```python
from build123d import *

# Parameters (mm, degrees)
SKETCH_1_R                   = 14
SKETCH_1_R_2                 = 2.75
EXTRUDE_1_DEPTH              = 27
CHAMFER_2_SIZE               = 1
HOLE_WIZARD_M5_4_D           = 5.5
HOLE_WIZARD_M5_4_CBORE_D     = 10
HOLE_WIZARD_M5_4_CBORE_DEPTH = 5.4
PATTERN_CIRCULAR_1_COUNT     = 4
SKETCH_15_R                  = 16
SKETCH_15_R_2                = 14
CUT_EXTRUDE_1_DEPTH          = 22
CHAMFER_3_SIZE               = 0.5


with BuildPart() as part:
    # 草圖1 → 填料-伸長1 (new body)
    with BuildSketch(Plane.XY):
        Polygon((55, 38), (70, 38), (70, 0), (0, 0), (0, 38), (15, 38), (15, 48), (55, 48), align=None)
        with Locations((35, 28)):
            Circle(SKETCH_1_R, mode=Mode.SUBTRACT)
        with Locations((8, 28)):
            Circle(SKETCH_1_R_2, mode=Mode.SUBTRACT)
        with Locations((62, 28)):
            Circle(SKETCH_1_R_2, mode=Mode.SUBTRACT)
        with Locations((8, 10)):
            Circle(SKETCH_1_R_2, mode=Mode.SUBTRACT)
        with Locations((62, 10)):
            Circle(SKETCH_1_R_2, mode=Mode.SUBTRACT)
    extrude(amount=-EXTRUDE_1_DEPTH)

    # 導角2
    chamfer_2_edges = [part.edges().sort_by_distance(p)[0] for p in [
        (15, 48, -13.5),
        (55, 48, -13.5),
    ]]
    chamfer(chamfer_2_edges, length=CHAMFER_2_SIZE)

    # M5 六角承窩頭蓋螺釘的柱孔4 (through all)
    with Locations(Plane(origin=(0, 38, 0), x_dir=(1, 0, 0), z_dir=(0, 1, 0))):
        with Locations((8, 21), (8, 6), (62, 21), (62, 6)):
            CounterBoreHole(HOLE_WIZARD_M5_4_D / 2, HOLE_WIZARD_M5_4_CBORE_D / 2, HOLE_WIZARD_M5_4_CBORE_DEPTH)

    # 草圖14 → M4 螺紋孔1 (revolve, cut)
    with BuildSketch(Plane(origin=(21.564971157, 41.435028843, 0), x_dir=(0, -1, 0), z_dir=(1, 0, 0))):
        Polygon((0, 0), (0, 12.991420021), (1.65, 12), (1.65, 0), align=None)
    hole_wizard_m4_1 = revolve(axis=Axis((21.564971157, 41.435028843, 6.35), (0, 0, -1)), mode=Mode.SUBTRACT)

    # 環狀複製排列1: M4 螺紋孔1 ×4 about axis
    pattern_circular_1_axis = Axis((35, 28, 0), (0, 0, 1))
    for i in range(1, PATTERN_CIRCULAR_1_COUNT):
        add(hole_wizard_m4_1.rotate(pattern_circular_1_axis, i * 360 / PATTERN_CIRCULAR_1_COUNT), mode=Mode.SUBTRACT)

    # 草圖15 → 除料-伸長1 (cut)
    with BuildSketch(Plane.XY):
        with Locations((35, 28)):
            Circle(SKETCH_15_R)
        with Locations((35, 28)):
            Circle(SKETCH_15_R_2, mode=Mode.SUBTRACT)
    extrude(amount=-CUT_EXTRUDE_1_DEPTH, mode=Mode.SUBTRACT)

    # 導角3
    chamfer_3_edges = [part.edges().sort_by_distance(p)[0] for p in [
        (70, 19, -27),
        (0, 19, 0),
        (62.5, 38, -27),
        (0, 38, -13.5),
        (70, 38, -13.5),
        (55, 42.5, -27),
        (7.5, 38, -27),
        (0, 19, -27),
        (35, 48, 0),
        (35, 48, -27),
        (15, 42.5, 0),
        (54.5, 47.5, 0),
        (15.5, 47.5, 0),
        (15, 42.5, -27),
        (54.5, 47.5, -27),
        (15.5, 47.5, -27),
        (7.5, 38, 0),
        (55, 42.5, 0),
        (62.5, 38, 0),
        (70, 19, 0),
    ]]
    chamfer(chamfer_3_edges, length=CHAMFER_3_SIZE)


solid = part.part
```
Geometry check sheet. Reference: the model listing, model coordinates, mm. A direction names the side the tool comes from. Give positions to 0.01 mm unless a question says otherwise; leave off trailing zeros. Order: outer loops, then holes, each group sorted by start corner. A loop starts at its lowest first (then second) coordinate and runs counter-clockwise, first axis right, second up. Notation, with made-up numbers: (31.25, 19.5) - (50.25, 19.5) arc R19 ccw to (50.25, 56.5) - close; hole circle Ø11 at (13, 61.25). An arc over 180 degrees is marked (long way). Answer in a Markdown table with one row per item. Add a question column.
Q1. Cross-section at C-C, the plane y = 3. Enter the section's corners in (x, z), then the cut area to 3 significant figures.
Q2. Cross-section at B-B, the plane y = 39. Enter the section's corners in (x, z), then the cut area to 3 significant figures.
Q3. Tool access check on faces 4 (the cylindrical face through (6.92, 35.34, -16.12)), 5 (the flat face through (70, 19, -13)), 6 (the flat face through (34.93, 13.85, -22)). Record the directions out of +Z, -Z, +X, -X, +Y, -Y that give a thin tool (end or side, any length) a straight path to the whole face; none if there is none.
Q4. Cross-section at D-D, the plane z = -19. Count the separate pieces of the cut face and the enclosed holes in it, then the cut area to 3 significant figures.
Q5. Material ranges on probe 1 along Y at (x, z) = (62, -17.75); probe 2 along Z at (x, y) = (8, 2.75); probe 3 along X at (y, z) = (10, -23.4), recorded low to high. Write a range as from..to.
Q6. Cross-section at A-A, the plane x = 35. Enter the section's corners in (y, z), then the cut area to 3 significant figures.
Q7. Gauge pin test, flat ends, axial feed: pin 1 (5 mm diameter, centred on x = 62, z = -21, fed in from +Y); pin 2 (10 mm diameter, centred on y = 44.5, z = -13.5, fed in from +X); pin 3 (16 mm diameter, centred on x = 6.5, z = -7.5, fed in from +Y); pin 4 (2 mm diameter, centred on x = 60, z = -5, fed in from +Y). Record the tip position at first contact, or that the pin passes through.
Q8. Mould release check, pull along Y, two halves, no side actions. Record for faces 1 (the cylindrical face through (19.917, 14.492, -5.916)), 2 (the flat face through (35.5, 13.5, -27)), 3 (the flat face through (35, 0, -13)): pulls with the +Y half, pulls with the -Y half, needs draft (parallel to the pull), parting line crosses it, or undercut.
Check values:
| question | item | result |
|---|---|---|
| 1 | outline | (0, -26.5) - (0.5, -27) - (69.5, -27) - (70, -26.5) - (70, -0.5) - (69.5, 0) - (0.5, 0) - (0, -0.5) - close; hole circle Ø5.5 at (8, -21); hole circle Ø5.5 at (8, -6); hole circle Ø5.5 at (62, -21); hole circle Ø5.5 at (62, -6) |
| 1 | area | 1,790 mm^2 |
| 2 | outline | (15, -26.5) - (15.5, -27) - (26.34, -27) - (26.34, -22) - (23.38, -22) - (23.38, 0) - (15.5, 0) - (15, -0.5) - close; (43.66, -27) - (54.5, -27) - (55, -26.5) - (55, -0.5) - (54.5, 0) - (46.62, 0) - (46.62, -22) - (43.66, -22) - close |
| 2 | area | 482 mm^2 |
| 3 | face 4 | +Y |
| 3 | face 5 | +Z, -Z, +X, +Y, -Y |
| 3 | face 6 | +Z |
| 4 | separate pieces | 3 |
| 4 | enclosed holes | 1 |
| 4 | area | 1,890 mm^2 |
| 5 | probe 1 | y = 0..7.25, 12.75..25.25, 30.75..32.6 |
| 5 | probe 2 | z = -27..-23.75, -18.25..-8.75, -3.25..0 |
| 5 | probe 3 | x = 0..5.25, 10.75..59.25, 64.75..70 |
| 6 | outline | (0, -27) - (14, -27) - (14, -22) - (12, -22) - (12, 0) - (0, 0) - close; (42, -27) - (47.5, -27) - (48, -26.5) - (48, -0.5) - (47.5, 0) - (44, 0) - (44, -22) - (42, -22) - close |
| 6 | area | 452 mm^2 |
| 7 | pin 1 | passes through |
| 7 | pin 2 | stops at x = 55 |
| 7 | pin 3 | stops at y = 38 |
| 7 | pin 4 | stops at y = 32.6 |
| 8 | face 1 | undercut |
| 8 | face 2 | needs draft |
| 8 | face 3 | pulls with the -Y half |
